Can you work these out from the model? Positions are in its coordinate system, mm. A direction names the side the tool comes from. Coordinates: 2 decimals unless noted, no trailing zeros. Order: outer loops, then holes, each group sorted by start corner. A loop starts at its lowest first (then second) coordinate and runs counter-clockwise, first axis right, second up. Notation, with made-up numbers: M 86.5,40 L 95.5,40 A26 cw 95.5,61 Z; hole C -36.5,19.25 d9. An arc over 180 degrees is marked long. Answer as CSV lines item,"result". Start each with the question number.
1. I need wall thicknesses on line 1 along X through (y, z) = (-25, 1); line 2 along Y through (x, z) = (22, 0); line 3 along Y through (x, z) = (22, -1). Which ranges of each line are inside material? Lowest first, please. Write a range as from..to.
2. If we section it at C-C (x = 27): List the corners of the cut face in (y, z) for me (3 decimals).
3. Will these pins go through, and if not, where does the flat tip stop? pin 1 (0.8 mm diameter, centred on y = -3.5, z = -2.5, fed in from +X) (3 decimals); pin 2 (8 mm diameter, centred on x = -24, z = 17.5, fed in from -Y); pin 3 (1.6 mm diameter, centred on x = 22, y = 22, fed in from +Z); pin 4 (2.5 mm diameter, centred on x = 22.7, y = -25.75, fed in from -Z).
4. On a 3-axis mill with a long thin cutter (end or side, diameter ignored), from which of +Z, -Z, +X, -X, +Y, -Y can I reach the whole of each face in a straight line? I mean faces 5 (the face through (-35.4, -23, 0.7)), 6 (the face through (0, 0, -2)), 7 (the face through (-13.574, -50.78, -0.028)). Say none if no direction works.
5. If we section it at B-B (y = -20.5): List the corners of the cut face in (x, z) for me (3 decimals).
6. If we mould it in two halves opening along X, with no side actions, what happens to faces 1 (the face through (13.496, -50.702, -0.028)), 2 (the face through (-47.62, -70.89, 30.13)), 3 (the face through (-15, -57, 0)), 4 (the face through (47.62, -96.88, -41.27))? For each: released by +X, released by -X, zero draft, split by the parting line, or undercut.
7. If we section it at A-A (x = 12.5): List the corners of the cut face in (y, z) for me (3 decimals).
8. If we section it at D-D (x = -13): List the corners of the cut face in (y, z) for me (3 decimals).
Autodesk Fusion 360 part; units mm, degrees
sketch "Sketch1" plane through (0, 0, 0) normal (0, 0, 1) x (1, 0, 0)
  line L0 (-51.9, 32.75) -> (51.9, 32.75)
  line L1 (51.9, 32.75) -> (51.9, -32.75)
  line L2 (51.9, -32.75) -> (-51.9, -32.75)
  line L3 (-51.9, -32.75) -> (-51.9, 32.75)
  point P0 (0, 32.75)
  point P1 (51.9, 0)
  dimension "d1" = 103.8
  dimension "d2" = 65.5
extrude "Extrude1" add sketch "Sketch1" along normal mid plane 4
sketch "Sketch2" plane through (0, 0, 2) normal (0, 0, 1) x (-1, 0, 0)
  line L0 (51.9, 32.75) -> (-51.9, 32.75)
  line L1 (-51.9, 32.75) -> (-51.9, -32.75)
  line L2 (-51.9, -32.75) -> (51.9, -32.75)
  line L3 (51.9, -32.75) -> (51.9, 32.75)
  point P0 (35.3, -23.25)
  point P1 (-22.7, -23.25)
  point P2 (35.3, 25.75)
  point P3 (-22.7, 25.75)
  dimension "d5" = 9.5
  dimension "d6" = 16.6
  dimension "d7" = 58
  dimension "d8" = 49
hole "Hole1" at (-35.3, 23.25, 2) at (22.7, 23.25, 2) at (22.7, -25.75, 2) at (-35.3, -25.75, 2) direction (0, 0, -1) diameter 2.9 depth 12 tip angle 118 counterbore diameter 5.5 counterbore depth 2.5
sketch "Sketch3" plane through (0, 0, -2) normal (0, 0, -1) x (1, 0, 0)
  circle A0 centre (22.7, 25.75) radius 1.45
  circle A1 centre (-35.3, -23.25) radius 1.45
  circle A2 centre (22.7, -23.25) radius 1.45
  circle A3 centre (-35.3, 25.75) radius 1.45
  line L0 (51.9, 32.75) -> (-51.9, 32.75)
  line L1 (-51.9, 32.75) -> (-51.9, -32.75)
  line L2 (-51.9, -32.75) -> (51.9, -32.75)
  line L3 (51.9, -32.75) -> (51.9, 32.75)
  line L4 (-48.775, 31.125) -> (50.275, 31.125)
  line L5 (50.275, 31.125) -> (50.275, -29.625)
  line L6 (50.275, -29.625) -> (-48.775, -29.625)
  line L7 (-48.775, -29.625) -> (-48.775, 31.125)
  line L8 (-46.775, 29.125) -> (48.275, 29.125)
  line L9 (48.275, 29.125) -> (48.275, -27.625)
  line L10 (48.275, -27.625) -> (-46.775, -27.625)
  line L11 (-46.775, -27.625) -> (-46.775, 29.125)
  point P0 (0.75, 31.125)
  point P1 (0.75, 29.125)
  point P2 (50.275, 0.75)
  point P3 (48.275, 0.75)
  dimension "d14" = 2
  dimension "d15" = 2
  dimension "d16" = 99.05
  dimension "d17" = 60.75
  dimension "d41" = 3.125
  dimension "d42" = 1.625
extrude "Extrude2" add sketch "Sketch3" along normal blind 1 contours L4 L5 L6 L7
sketch "Sketch5" plane through (0, 0, 2) normal (0, 0, 1) x (-1, 0, 0)
  circle A0 centre (-22.7, 25.75) radius 2.75
  circle A1 centre (35.3, -23.25) radius 2.75
  circle A2 centre (-22.7, -23.25) radius 2.75
  circle A3 centre (35.3, 25.75) radius 2.75
  line L0 (51.9, 32.75) -> (-51.9, 32.75)
  line L1 (-51.9, 32.75) -> (-51.9, -32.75)
  line L2 (-51.9, -32.75) -> (51.9, -32.75)
  line L3 (51.9, -32.75) -> (51.9, 32.75)
  line L4 (51.9, 32.75) -> (-51.9, 32.75)
  line L5 (-51.9, 32.75) -> (-51.9, 82.75)
  line L6 (-51.9, 82.75) -> (51.9, 82.75)
  line L7 (51.9, 82.75) -> (51.9, 32.75)
  dimension "d20" = 50
extrude "Extrude3" add sketch "Sketch5" against normal up to surface (4 mm away) contours L0 L4 L5 L6 L7
sketch "Sketch7" plane through (-51.9, 0, 0) normal (-1, 0, 0) x (0, -1, 0)
  line L0 (82.75, 2) -> (-32.75, 2)
  line L1 (-32.75, 2) -> (-32.75, -2)
  line L2 (-32.75, -2) -> (82.75, -2)
  line L3 (82.75, -2) -> (82.75, 2)
  line L4 (82.75, 2) -> (99.851, -44.9846)
  line L5 (99.851, -44.9846) -> (97.0319, -46.0107)
  line L6 (97.0319, -46.0107) -> (81.0133, -2)
  line L7 (82.75, 2) -> (70.7793, 34.8892)
  line L8 (70.7793, 34.8892) -> (67.9602, 33.8632)
  line L9 (67.9602, 33.8632) -> (81.0133, -2)
  dimension "d23" = 70
  dimension "d24" = 50
  dimension "d27" = 3
  dimension "d28" = 35
extrude "Extrude4" add sketch "Sketch7" against normal up to surface (103.8 mm away) contours L2 L3 L4 L5 L6 | L0 L7 L8 L9
fillet "Fillet1" radius 15 4 edges at (-51.9, -69.3698, 34.3762) (51.9, -69.3698, 34.3762) (51.9, -98.4415, -45.4977) (-51.9, -98.4415, -45.4977)
fillet "Fillet2" radius 10 2 edges at (0, -81.0133, -2) (0, -79.5575, 2)
sketch "Sketch8" plane through (0, 0, 2) normal (0, 0, 1) x (-1, 0, 0)
  line L0 (51.9, 65.276) -> (-51.9, 65.276)
  line L1 (-51.9, 65.276) -> (-51.9, -32.75)
  line L2 (-51.9, -32.75) -> (51.9, -32.75)
  line L3 (51.9, -32.75) -> (51.9, 65.276)
  circle A0 centre (-22.7, 25.75) radius 2.75
  circle A1 centre (35.3, -23.25) radius 2.75
  circle A2 centre (-22.7, -23.25) radius 2.75
  circle A3 centre (35.3, 25.75) radius 2.75
  line L4 (15, 49.276) -> (-15, 49.276)
  line L5 (-15, 49.276) -> (-15, 64.276)
  line L6 (-15, 64.276) -> (15, 64.276)
  line L7 (15, 64.276) -> (15, 49.276)
  point P0 (0, 49.276)
  dimension "d33" = 1
  dimension "d34" = 15
  dimension "d35" = 30
extrude "Extrude5" cut sketch "Sketch8" against normal up to surface (4 mm away) contours L4 L5 L6 L7
fillet "Fillet3" radius 5 4 edges at (-15, -64.276, 0) (15, -64.276, 0) (15, -49.276, 0) (-15, -49.276, 0)
equation "d15 = d14"
equation "d16 = 99.30 mm - 0.25 mm"
equation "d17 = 61.00 mm - 0.25 mm"
equation "d41 = 3 mm + ( 0.25 / 2 ) * 1 mm"
equation "d42 = 1.5 mm + ( 0.25 / 2 ) * 1 mm"
Solved:
1,line 1,"-51.9..-37.95, -32.65..20.05, 25.35..51.9"
1,line 2,"-83.48..-28.41, -23.09..20.59, 25.91..32.75"
1,line 3,"-83.84..-27.02, -24.48..21.98, 24.52..32.75"
2,outline,"M -99.851,-44.985 L -97.032,-46.011 L -83.408,-8.58 A10 cw -74.011,-2 L -31.125,-2 L -31.125,-3 L -29.125,-3 L -29.125,-2 L 27.625,-2 L 27.625,-3 L 29.625,-3 L 29.625,-2 L 32.75,-2 L 32.75,2 L -65.276,2 A10 cw -74.673,15.42 L -67.96,33.863 L -70.779,34.889 L -82.75,2 Z"
3,pin 1,"x = 50.275"
3,pin 2,"y = -78.56"
3,pin 3,"z = -0.5"
3,pin 4,"through"
4,face 5,"+Z"
4,face 6,"-Z"
4,face 7,"+Z, -Z"
5,outline,"M -51.9,-2 L -48.775,-2 L -48.775,-3 L -46.775,-3 L -46.775,-2 L 48.275,-2 L 48.275,-3 L 50.275,-3 L 50.275,-2 L 51.9,-2 L 51.9,2 L -51.9,2 Z"
6,face 1,"undercut"
6,face 2,"released by -X"
6,face 3,"undercut"
6,face 4,"released by +X"
7,outline,"M -99.851,-44.985 L -97.032,-46.011 L -83.408,-8.58 A10 cw -74.011,-2 L -63.606,-2 L -63.606,2 L -65.276,2 A10 cw -74.673,15.42 L -67.96,33.863 L -70.779,34.889 L -82.75,2 Z; M -49.946,-2 L -31.125,-2 L -31.125,-3 L -29.125,-3 L -29.125,-2 L 27.625,-2 L 27.625,-3 L 29.625,-3 L 29.625,-2 L 32.75,-2 L 32.75,2 L -49.946,2 Z"
8,outline,"M -99.851,-44.985 L -97.032,-46.011 L -83.408,-8.58 A10 cw -74.011,-2 L -63.276,-2 L -63.276,2 L -65.276,2 A10 cw -74.673,15.42 L -67.96,33.863 L -70.779,34.889 L -82.75,2 Z; M -50.276,-2 L -31.125,-2 L -31.125,-3 L -29.125,-3 L -29.125,-2 L 27.625,-2 L 27.625,-3 L 29.625,-3 L 29.625,-2 L 32.75,-2 L 32.75,2 L -50.276,2 Z"
